Part model, mm, in its own coordinate system. Round coordinates to 2 decimals unless told otherwise and drop trailing zeros. Loops run counter-clockwise (first coordinate to the right, second up) from the corner with the lowest first, then second, coordinate; pieces in that order, holes last.
(1) Mould opens along Y. For faces 1 (the face through (1.521, 326.084, -626.935)), 2 (the face through (3, 511, -547)), 3 (the face through (1.52, 411.44, -604.75)) say: +Y half, -Y half, draft (parallel to the pull), parting line (faces both ways), or undercut.
(2) Cut at A-A on x = 0.55. Count the separate pieces of the cut face and the enclosed holes in it, then the cut area to 3 significant figures.
(3) Cut at B-B on z = -526. List the corners of the cut face in (x, y), then the cut area to 3 significant figures.
(4) Probe probe 1 along Y at (x, z) = (1.95, -484); probe 2 along Y at (x, z) = (1.2, -608); probe 3 along Z at (x, y) = (2.25, 602). List the from-to ranges inside material, lowest first.
(5) Cut at C-C on y = 628. List the corners of the cut face in (x, z), then the cut area to 3 significant figures.
(6) Flat gauge pins, fed straight in: pin 1 (7 mm diameter, centred on y = 673.98, z = -606.95, fed in from +X); pin 2 (1.5 mm diameter, centred on x = 2, z = -567, fed in from -Y); pin 3 (1 mm diameter, centred on x = 2, z = -518.5, fed in from +Y). Where does each tip first touch, or does it go through?
from build123d import *

# Parameters (mm, degrees)
BOSS_EXTRUDE1_DEPTH = 3
CUT_EXTRUDE1_REACH  = 5
SKETCH3_R           = 3
CUT_EXTRUDE2_REACH  = 5
SKETCH4_R           = 5
FILLET1_R           = 10


with BuildPart() as part:
    # Sketch1 → Boss-Extrude1 (new body)
    with BuildSketch(Plane(origin=(0, 0, 0), x_dir=(0, 0, -1), z_dir=(1, 0, 0))):
        Polygon((459.131022606, 411.733722484), (459.131022606, 597.849507888), (631.946459815, 700.452034157), (631.946459815, 317.945389168), align=None)
    extrude(amount=BOSS_EXTRUDE1_DEPTH)

    # Sketch3 → Cut-Extrude1 (cut, up to next)
    with BuildSketch(Plane(origin=(3, 0, 0), x_dir=(0, 0, -1), z_dir=(1, 0, 0)), mode=Mode.PRIVATE) as cut_extrude1_sk1:
        with Locations((516.660188982, 620.375565005)):
            Circle(SKETCH3_R)
    cut_extrude1_tool1 = extrude(cut_extrude1_sk1.sketch, amount=-CUT_EXTRUDE1_REACH, mode=Mode.PRIVATE) & part.part
    add(cut_extrude1_tool1.solids().sort_by_distance((3, 620.375565, -516.660189))[0], mode=Mode.SUBTRACT)
    # Sketch3 → Cut-Extrude1 (cut, up to next)
    with BuildSketch(Plane(origin=(3, 0, 0), x_dir=(0, 0, -1), z_dir=(1, 0, 0)), mode=Mode.PRIVATE) as cut_extrude1_sk2:
        with Locations((546.755612593, 638.243566507)):
            Circle(SKETCH3_R)
    cut_extrude1_tool2 = extrude(cut_extrude1_sk2.sketch, amount=-CUT_EXTRUDE1_REACH, mode=Mode.PRIVATE) & part.part
    add(cut_extrude1_tool2.solids().sort_by_distance((3, 638.243567, -546.755613))[0], mode=Mode.SUBTRACT)
    # Sketch3 → Cut-Extrude1 (cut, up to next)
    with BuildSketch(Plane(origin=(3, 0, 0), x_dir=(0, 0, -1), z_dir=(1, 0, 0)), mode=Mode.PRIVATE) as cut_extrude1_sk3:
        with Locations((576.851036204, 656.111568009)):
            Circle(SKETCH3_R)
    cut_extrude1_tool3 = extrude(cut_extrude1_sk3.sketch, amount=-CUT_EXTRUDE1_REACH, mode=Mode.PRIVATE) & part.part
    add(cut_extrude1_tool3.solids().sort_by_distance((3, 656.111568, -576.851036))[0], mode=Mode.SUBTRACT)
    # Sketch3 → Cut-Extrude1 (cut, up to next)
    with BuildSketch(Plane(origin=(3, 0, 0), x_dir=(0, 0, -1), z_dir=(1, 0, 0)), mode=Mode.PRIVATE) as cut_extrude1_sk4:
        with Locations((514.66108198, 392.974861297)):
            Circle(SKETCH3_R)
    cut_extrude1_tool4 = extrude(cut_extrude1_sk4.sketch, amount=-CUT_EXTRUDE1_REACH, mode=Mode.PRIVATE) & part.part
    add(cut_extrude1_tool4.solids().sort_by_distance((3, 392.974861, -514.661082))[0], mode=Mode.SUBTRACT)
    # Sketch3 → Cut-Extrude1 (cut, up to next)
    with BuildSketch(Plane(origin=(3, 0, 0), x_dir=(0, 0, -1), z_dir=(1, 0, 0)), mode=Mode.PRIVATE) as cut_extrude1_sk5:
        with Locations((545.422874592, 376.280188034)):
            Circle(SKETCH3_R)
    cut_extrude1_tool5 = extrude(cut_extrude1_sk5.sketch, amount=-CUT_EXTRUDE1_REACH, mode=Mode.PRIVATE) & part.part
    add(cut_extrude1_tool5.solids().sort_by_distance((3, 376.280188, -545.422875))[0], mode=Mode.SUBTRACT)
    # Sketch3 → Cut-Extrude1 (cut, up to next)
    with BuildSketch(Plane(origin=(3, 0, 0), x_dir=(0, 0, -1), z_dir=(1, 0, 0)), mode=Mode.PRIVATE) as cut_extrude1_sk6:
        with Locations((576.184667203, 359.585514772)):
            Circle(SKETCH3_R)
    cut_extrude1_tool6 = extrude(cut_extrude1_sk6.sketch, amount=-CUT_EXTRUDE1_REACH, mode=Mode.PRIVATE) & part.part
    add(cut_extrude1_tool6.solids().sort_by_distance((3, 359.585515, -576.184667))[0], mode=Mode.SUBTRACT)
    # Sketch3 → Cut-Extrude1 (cut, up to next)
    with BuildSketch(Plane(origin=(3, 0, 0), x_dir=(0, 0, -1), z_dir=(1, 0, 0)), mode=Mode.PRIVATE) as cut_extrude1_sk7:
        with Locations((486.564765371, 602.507563503)):
            Circle(SKETCH3_R)
    cut_extrude1_tool7 = extrude(cut_extrude1_sk7.sketch, amount=-CUT_EXTRUDE1_REACH, mode=Mode.PRIVATE) & part.part
    add(cut_extrude1_tool7.solids().sort_by_distance((3, 602.507564, -486.564765))[0], mode=Mode.SUBTRACT)
    # Sketch3 → Cut-Extrude1 (cut, up to next)
    with BuildSketch(Plane(origin=(3, 0, 0), x_dir=(0, 0, -1), z_dir=(1, 0, 0)), mode=Mode.PRIVATE) as cut_extrude1_sk8:
        with Locations((606.946459815, 673.979569511)):
            Circle(SKETCH3_R)
    cut_extrude1_tool8 = extrude(cut_extrude1_sk8.sketch, amount=-CUT_EXTRUDE1_REACH, mode=Mode.PRIVATE) & part.part
    add(cut_extrude1_tool8.solids().sort_by_distance((3, 673.97957, -606.94646))[0], mode=Mode.SUBTRACT)
    # Sketch3 → Cut-Extrude1 (cut, up to next)
    with BuildSketch(Plane(origin=(3, 0, 0), x_dir=(0, 0, -1), z_dir=(1, 0, 0)), mode=Mode.PRIVATE) as cut_extrude1_sk9:
        with Locations((483.899289369, 409.669534559)):
            Circle(SKETCH3_R)
    cut_extrude1_tool9 = extrude(cut_extrude1_sk9.sketch, amount=-CUT_EXTRUDE1_REACH, mode=Mode.PRIVATE) & part.part
    add(cut_extrude1_tool9.solids().sort_by_distance((3, 409.669535, -483.899289))[0], mode=Mode.SUBTRACT)
    # Sketch3 → Cut-Extrude1 (cut, up to next)
    with BuildSketch(Plane(origin=(3, 0, 0), x_dir=(0, 0, -1), z_dir=(1, 0, 0)), mode=Mode.PRIVATE) as cut_extrude1_sk10:
        with Locations((606.946459815, 342.89084151)):
            Circle(SKETCH3_R)
    cut_extrude1_tool10 = extrude(cut_extrude1_sk10.sketch, amount=-CUT_EXTRUDE1_REACH, mode=Mode.PRIVATE) & part.part
    add(cut_extrude1_tool10.solids().sort_by_distance((3, 342.890842, -606.94646))[0], mode=Mode.SUBTRACT)

    # Sketch4 → Cut-Extrude2 (cut, up to next)
    with BuildSketch(Plane(origin=(3, 0, 0), x_dir=(0, 0, -1), z_dir=(1, 0, 0)), mode=Mode.PRIVATE) as cut_extrude2_sk1:
        with Locations((602.36530116, 596.288363913)):
            Circle(SKETCH4_R)
    cut_extrude2_tool1 = extrude(cut_extrude2_sk1.sketch, amount=-CUT_EXTRUDE2_REACH, mode=Mode.PRIVATE) & part.part
    add(cut_extrude2_tool1.solids().sort_by_distance((3, 596.288364, -602.365301))[0], mode=Mode.SUBTRACT)
    # Sketch4 → Cut-Extrude2 (cut, up to next)
    with BuildSketch(Plane(origin=(3, 0, 0), x_dir=(0, 0, -1), z_dir=(1, 0, 0)), mode=Mode.PRIVATE) as cut_extrude2_sk2:
        with Locations((603.522472038, 536.299523655)):
            Circle(SKETCH4_R)
    cut_extrude2_tool2 = extrude(cut_extrude2_sk2.sketch, amount=-CUT_EXTRUDE2_REACH, mode=Mode.PRIVATE) & part.part
    add(cut_extrude2_tool2.solids().sort_by_distance((3, 536.299524, -603.522472))[0], mode=Mode.SUBTRACT)
    # Sketch4 → Cut-Extrude2 (cut, up to next)
    with BuildSketch(Plane(origin=(3, 0, 0), x_dir=(0, 0, -1), z_dir=(1, 0, 0)), mode=Mode.PRIVATE) as cut_extrude2_sk3:
        with Locations((604.679642916, 476.310683396)):
            Circle(SKETCH4_R)
    cut_extrude2_tool3 = extrude(cut_extrude2_sk3.sketch, amount=-CUT_EXTRUDE2_REACH, mode=Mode.PRIVATE) & part.part
    add(cut_extrude2_tool3.solids().sort_by_distance((3, 476.310683, -604.679643))[0], mode=Mode.SUBTRACT)
    # Sketch4 → Cut-Extrude2 (cut, up to next)
    with BuildSketch(Plane(origin=(3, 0, 0), x_dir=(0, 0, -1), z_dir=(1, 0, 0)), mode=Mode.PRIVATE) as cut_extrude2_sk4:
        with Locations((605.836813794, 416.321843138)):
            Circle(SKETCH4_R)
    cut_extrude2_tool4 = extrude(cut_extrude2_sk4.sketch, amount=-CUT_EXTRUDE2_REACH, mode=Mode.PRIVATE) & part.part
    add(cut_extrude2_tool4.solids().sort_by_distance((3, 416.321843, -605.836814))[0], mode=Mode.SUBTRACT)
    # Sketch4 → Cut-Extrude2 (cut, up to next)
    with BuildSketch(Plane(origin=(3, 0, 0), x_dir=(0, 0, -1), z_dir=(1, 0, 0)), mode=Mode.PRIVATE) as cut_extrude2_sk5:
        with Locations((502.953007582, 564.856704632)):
            Circle(SKETCH4_R)
    cut_extrude2_tool5 = extrude(cut_extrude2_sk5.sketch, amount=-CUT_EXTRUDE2_REACH, mode=Mode.PRIVATE) & part.part
    add(cut_extrude2_tool5.solids().sort_by_distance((3, 564.856705, -502.953008))[0], mode=Mode.SUBTRACT)
    # Sketch4 → Cut-Extrude2 (cut, up to next)
    with BuildSketch(Plane(origin=(3, 0, 0), x_dir=(0, 0, -1), z_dir=(1, 0, 0)), mode=Mode.PRIVATE) as cut_extrude2_sk6:
        with Locations((504.110178459, 504.867864374)):
            Circle(SKETCH4_R)
    cut_extrude2_tool6 = extrude(cut_extrude2_sk6.sketch, amount=-CUT_EXTRUDE2_REACH, mode=Mode.PRIVATE) & part.part
    add(cut_extrude2_tool6.solids().sort_by_distance((3, 504.867864, -504.110178))[0], mode=Mode.SUBTRACT)
    # Sketch4 → Cut-Extrude2 (cut, up to next)
    with BuildSketch(Plane(origin=(3, 0, 0), x_dir=(0, 0, -1), z_dir=(1, 0, 0)), mode=Mode.PRIVATE) as cut_extrude2_sk7:
        with Locations((505.267349337, 444.879024115)):
            Circle(SKETCH4_R)
    cut_extrude2_tool7 = extrude(cut_extrude2_sk7.sketch, amount=-CUT_EXTRUDE2_REACH, mode=Mode.PRIVATE) & part.part
    add(cut_extrude2_tool7.solids().sort_by_distance((3, 444.879024, -505.267349))[0], mode=Mode.SUBTRACT)

    # Fillet1
    fillet1_edges = [part.edges().sort_by_distance(p)[0] for p in [
        (1.5, 411.733722484, -459.131022606),
        (1.5, 597.849507888, -459.131022606),
        (1.5, 700.452034157, -631.946459815),
        (1.5, 317.945389168, -631.946459815),
    ]]
    fillet(fillet1_edges, radius=FILLET1_R)


solid = part.part
Final values:
1. face 1: -Y half
1. face 2: draft
1. face 3: undercut
2. separate pieces: 1
2. enclosed holes: 17
2. area: 48,200 mm2
3. outline: (0, 375.44) - (3, 375.44) - (3, 637.55) - (0, 637.55) - close
3. area: 786 mm2
4. probe 1: y = 398.24 to 406.67, 412.67 to 600.95, 604.06 to 612.61
4. probe 2: y = 330.94 to 340.08, 345.7 to 411.81, 420.83 to 472.57, 480.05 to 534.07, 538.52 to 671.17, 676.79 to 686.23
4. probe 3: z = -631.95 to -489.52, -483.61 to -466.12
5. outline: (0, -631.95) - (3, -631.95) - (3, -509.91) - (0, -509.91) - close
5. area: 366 mm2
6. pin 1: stops at x = 3
6. pin 2: stops at y = 352.79
6. pin 3: stops at y = 633.39
